from build123d import *

# Parameters (mm, degrees)
F1_DEPTH  = 4
F2_DEPTH  = 12
F7_W      = 2
F7_H      = 2
F7_H_2    = 1.95
F8_DEPTH  = 4
F9_DEPTH  = 8
F11_DEPTH = 4


with BuildPart() as f1:
    # F0 (on Right) → F1 (new body)
    with BuildSketch(Plane.YZ):
        with BuildLine():
            Line((4.95, 0), (4.95, 6.25))
            Line((4.95, 6.25), (1.95, 6.25))
            Line((1.95, 6.25), (0, 6.25))
            Line((0, 6.25), (-1.95, 6.25))
            Line((-1.95, 6.25), (-4.95, 6.25))
            Line((-4.95, 6.25), (-4.95, -2.25))
            Line((-4.95, -2.25), (-3, -2.25))
            ThreePointArc((-3, -2.25), (-1.1858541226, 3.5575623677), (3.75, 0))
            Line((3.75, 0), (4.95, 0))
        make_face()
        Polygon((-4.95, 6.25), (-1.95, 6.25), (-1.95, 11.25), (-1.95, 16.25), (-4.95, 16.25), align=None)
        Polygon((1.95, 6.25), (4.95, 6.25), (4.95, 16.25), (1.95, 16.25), (1.95, 11.25), align=None)
        with BuildLine():
            Line((4.95, -6.25), (4.95, -2.25))
            Line((4.95, -2.25), (3, -2.25))
            ThreePointArc((3, -2.25), (0, -3.75), (-3, -2.25))
            Line((-3, -2.25), (-4.95, -2.25))
            Line((-4.95, -2.25), (-4.95, -6.25))
            Line((-4.95, -6.25), (4.95, -6.25))
        make_face()
        with BuildLine():
            Line((4.95, -2.25), (4.95, 0))
            Line((4.95, 0), (3.75, 0))
            ThreePointArc((3.75, 0), (3.5575623677, -1.1858541226), (3, -2.25))
            Line((3, -2.25), (4.95, -2.25))
        make_face()
        with BuildLine():
            ThreePointArc((-3, -2.25), (0, -3.75), (3, -2.25))
            Line((3, -2.25), (0, -2.25))
            Line((0, -2.25), (-3, -2.25))
        make_face()
        with BuildLine():
            Line((2.25, 0), (3.75, 0))
            ThreePointArc((3.75, 0), (-1.1858541226, 3.5575623677), (-3, -2.25))
            Line((-3, -2.25), (0, -2.25))
            ThreePointArc((0, -2.25), (-1.5909902577, 1.5909902577), (2.25, 0))
        make_face()
        with BuildLine():
            ThreePointArc((3, -2.25), (3.5575623677, -1.1858541226), (3.75, 0))
            Line((3.75, 0), (2.25, 0))
            ThreePointArc((2.25, 0), (1.5909902577, -1.5909902577), (0, -2.25))
            Line((0, -2.25), (3, -2.25))
        make_face()
        Polygon((-1.95, 6.25), (0, 6.25), (-1.95, 11.25), align=None)
        Polygon((0, 6.25), (1.95, 6.25), (1.95, 11.25), align=None)
    extrude(amount=-F1_DEPTH)

    # F4: F1 across plane


with BuildPart() as f2:
    # F0 (on Right) → F2 (new body)
    with BuildSketch(Plane.YZ):
        with BuildLine():
            Line((4.95, -6.25), (4.95, -2.25))
            Line((4.95, -2.25), (3, -2.25))
            ThreePointArc((3, -2.25), (0, -3.75), (-3, -2.25))
            Line((-3, -2.25), (-4.95, -2.25))
            Line((-4.95, -2.25), (-4.95, -6.25))
            Line((-4.95, -6.25), (4.95, -6.25))
        make_face()
    extrude(amount=F2_DEPTH)


with BuildPart() as f1_1:
    add(f1.part)
    add(f1.part.mirror(Plane(origin=(-2, 3.45, 16.25), x_dir=(1, 0, 0), z_dir=(0, 0, 1))))


with BuildPart() as f6_1:
    # F6: instance of F1
    add(f1_1.part.mirror(Plane(origin=(0, 35, 0), x_dir=(-1, 0, 0), z_dir=(0, 1, 0))))


with BuildPart() as f6_2:
    # F6: instance of F2
    add(f2.part.mirror(Plane(origin=(0, 35, 0), x_dir=(-1, 0, 0), z_dir=(0, 1, 0))))


with BuildPart() as f8:
    # F7 (on face) → F8 (new body)
    with BuildSketch(Plane.XY.offset(-2.25)):
        Polygon((2, 28.35), (2, 4.95), (12, 4.95), (12, 28.35), (4, 28.35), align=None)
        Polygon((4, 30.35), (4, 28.35), (12, 28.35), (24, 28.35), (24, 30.35), align=None)
        with Locations((3, 29.35)):
            Rectangle(F7_W, F7_H)
        with Locations((3, 31.325)):
            Rectangle(F7_W, F7_H_2)
        with Locations((3, 38.675)):
            Rectangle(F7_W, F7_H_2)
        with Locations((3, 40.65)):
            Rectangle(F7_W, F7_H)
        Polygon((4, 39.65), (24, 39.65), (24, 41.65), (12, 41.65), (4, 41.65), align=None)
        Polygon((2, 65.05), (2, 41.65), (4, 41.65), (12, 41.65), (12, 65.05), align=None)
        Polygon((4, 32.3), (4, 30.35), (24, 30.35), (24, 39.65), (4, 39.65), (4, 37.7), align=None)
        Polygon((2, 35), (2, 32.3), (4, 32.3), (4, 37.7), (2, 37.7), align=None)
    extrude(amount=-F8_DEPTH)


with BuildPart() as f1_2:
    add(f1_1.part)

    add(f2.part)  # F9 merges F2

    add(f6_1.part)  # F9 merges F6_1

    add(f6_2.part)  # F9 merges F6_2

    add(f8.part)  # F9 merges F8
    # F7 (on face) → F9 (join)
    with BuildSketch(Plane.XY.offset(-2.25)):
        Polygon((4, 39.65), (24, 39.65), (24, 41.65), (12, 41.65), (4, 41.65), align=None)
        with Locations((3, 40.65)):
            Rectangle(F7_W, F7_H)
        with Locations((3, 38.675)):
            Rectangle(F7_W, F7_H_2)
        with Locations((3, 31.325)):
            Rectangle(F7_W, F7_H_2)
        with Locations((3, 29.35)):
            Rectangle(F7_W, F7_H)
        Polygon((4, 30.35), (4, 28.35), (12, 28.35), (24, 28.35), (24, 30.35), align=None)
    extrude(amount=F9_DEPTH)

    # F10 (on Right) → F11 (cut)
    with BuildSketch(Plane.YZ):
        with BuildLine():
            ThreePointArc((0, 34.75), (0.8610377228, 34.5787289482), (1.5909902577, 34.0909902577))
            Line((1.5909902577, 34.0909902577), (0, 35.6819805153))
            Line((0, 35.6819805153), (-1.5909902577, 34.0909902577))
            ThreePointArc((-1.5909902577, 34.0909902577), (-0.8610377228, 34.5787289482), (0, 34.75))
        make_face()
        with BuildLine():
            ThreePointArc((-1.5909902577, 1.5909902577), (-0.8610377228, 2.0787289482), (0, 2.25))
            ThreePointArc((0, 2.25), (0.8610377228, 2.0787289482), (1.5909902577, 1.5909902577))
            Line((1.5909902577, 1.5909902577), (0, 3.1819805153))
            Line((0, 3.1819805153), (-1.5909902577, 1.5909902577))
        make_face()
        with BuildLine():
            ThreePointArc((70, 2.25), (70.8610377228, 2.0787289482), (71.5909902577, 1.5909902577))
            Line((71.5909902577, 1.5909902577), (70, 3.1819805153))
            Line((70, 3.1819805153), (68.4090097423, 1.5909902577))
            ThreePointArc((68.4090097423, 1.5909902577), (69.1389622772, 2.0787289482), (70, 2.25))
        make_face()
        with BuildLine():
            ThreePointArc((70, 34.75), (70.8610377228, 34.5787289482), (71.5909902577, 34.0909902577))
            Line((71.5909902577, 34.0909902577), (70, 35.6819805153))
            Line((70, 35.6819805153), (68.4090097423, 34.0909902577))
            ThreePointArc((68.4090097423, 34.0909902577), (69.1389622772, 34.5787289482), (70, 34.75))
        make_face()
    extrude(amount=-F11_DEPTH, mode=Mode.SUBTRACT)


solid = f1_2.part
Here's how the part is built. I have some questions about the finished solid (model axes, mm). A direction names the side the tool comes from. Coordinates: 2 decimals unless noted, no trailing zeros. Order: outer loops, then holes, each group sorted by start corner. A loop starts at its lowest first (then second) coordinate and runs counter-clockwise, first axis right, second up. Notation, with made-up numbers: M 12.5,-2.5 L 62.5,-2.5 A20 ccw 62.5,1.5 Z; hole C 67.25,33 d11. An arc over 180 degrees is marked long. Answer as CSV lines item,"result". Start each with the question number.
1. I need wall thicknesses on line 1 (Y direction, x = -2.1, z = 32.5); line 2 (Y direction, x = 8.25, z = 5); line 3 (Y direction, x = -1.25, z = 23). Which ranges of each line are inside material? Lowest first, please. Write a range as [from, to].
2. We'd pull the mould along Z, two halves only. Please class faces 1 (the flat face through (2, 35, -3)), 2 (the cylindrical face through (5.92, 69.95, -3.75)), 3 (the flat face through (-1.972, 0.807, 34.875)): released by +Z, released by -Z, zero draft, split by the parting line, or undercut.
3. I want a section at A-A, the plane z = 28.5. Write out the boundary of the cut face in (x, y), and give its area (3 significant figures).
4. I want a section at D-D, the plane y = 11. Write out the boundary of the cut face in (x, z), and give its area (3 significant figures).
5. I want a section at B-B, the plane z = 13. Write out the boundary of the cut face in (x, y).
6. I want a section at C-C, the plane x = 10. Write out the boundary of the cut face in (y, z).
7. For pin 1 (3 mm diameter, centred on x = 14, y = 45, fed in from +Z) (3 decimals); pin 2 (0.6 mm diameter, centred on y = 38.5, z = 2, fed in from +X); pin 3 (10 mm diameter, centred on x = 18, y = 33, fed in from +Z); pin 4 (13 mm diameter, centred on y = 26, z = 2, fed in from -X), each with a flat end and sliding along its axis, tell me the tip position at first contact or that it passes through.
8. On a 3-axis mill with a long thin cutter (end or side, diameter ignored), from which of +Z, -Z, +X, -X, +Y, -Y can I reach the whole of each face in a straight line? I mean faces 4 (the flat face through (-2, 65.05, 16)), 5 (the flat face through (-2, 70, 38.75)), 6 (the flat face through (3, 37.7, 2)), 7 (the flat face through (-0.2, 74.95, 13)), 8 (the flat face through (-1.972, 70.807, 34.875)). Say none if no direction works.
Recorded:
1,line 1,"y = [-4.95, -2.25], [2.25, 4.95], [65.05, 67.75], [72.25, 74.95]"
1,line 2,"y = [28.35, 30.35], [39.65, 41.65]"
1,line 3,"y = [-4.95, -1.27], [1.27, 4.95], [65.05, 68.73], [71.27, 74.95]"
2,face 1,"zero draft"
2,face 2,"released by +Z"
2,face 3,"undercut"
3,outline,"M -4,-4.95 L 0,-4.95 L 0,4.95 L -4,4.95 Z; M -4,65.05 L 0,65.05 L 0,74.95 L -4,74.95 Z"
3,area,"79.2 mm2"
4,outline,"M 2,-6.25 L 12,-6.25 L 12,-2.25 L 2,-2.25 Z"
4,area,"40.0 mm2"
5,outline,"M -4,-4.95 L 0,-4.95 L 0,-1.95 L -4,-1.95 Z; M -4,1.95 L 0,1.95 L 0,4.95 L -4,4.95 Z; M -4,65.05 L 0,65.05 L 0,68.05 L -4,68.05 Z; M -4,71.95 L 0,71.95 L 0,74.95 L -4,74.95 Z"
6,outline,"M -4.95,-6.25 L 74.95,-6.25 L 74.95,-2.25 L 73,-2.25 A3.75 cw 67,-2.25 L 41.65,-2.25 L 41.65,5.75 L 39.65,5.75 L 39.65,-2.25 L 30.35,-2.25 L 30.35,5.75 L 28.35,5.75 L 28.35,-2.25 L 3,-2.25 A3.75 cw -3,-2.25 L -4.95,-2.25 Z"
7,pin 1,"passes through"
7,pin 2,"stops at x = 4"
7,pin 3,"stops at z = 5.75"
7,pin 4,"stops at x = 2"
8,face 4,"+Z, -Z, -X"
8,face 5,"+Z, +X, -X, +Y, -Y"
8,face 6,"+Z, +X, -X"
8,face 7,"+Z, -Z, +X, -X, +Y"
8,face 8,"+X, -X"
